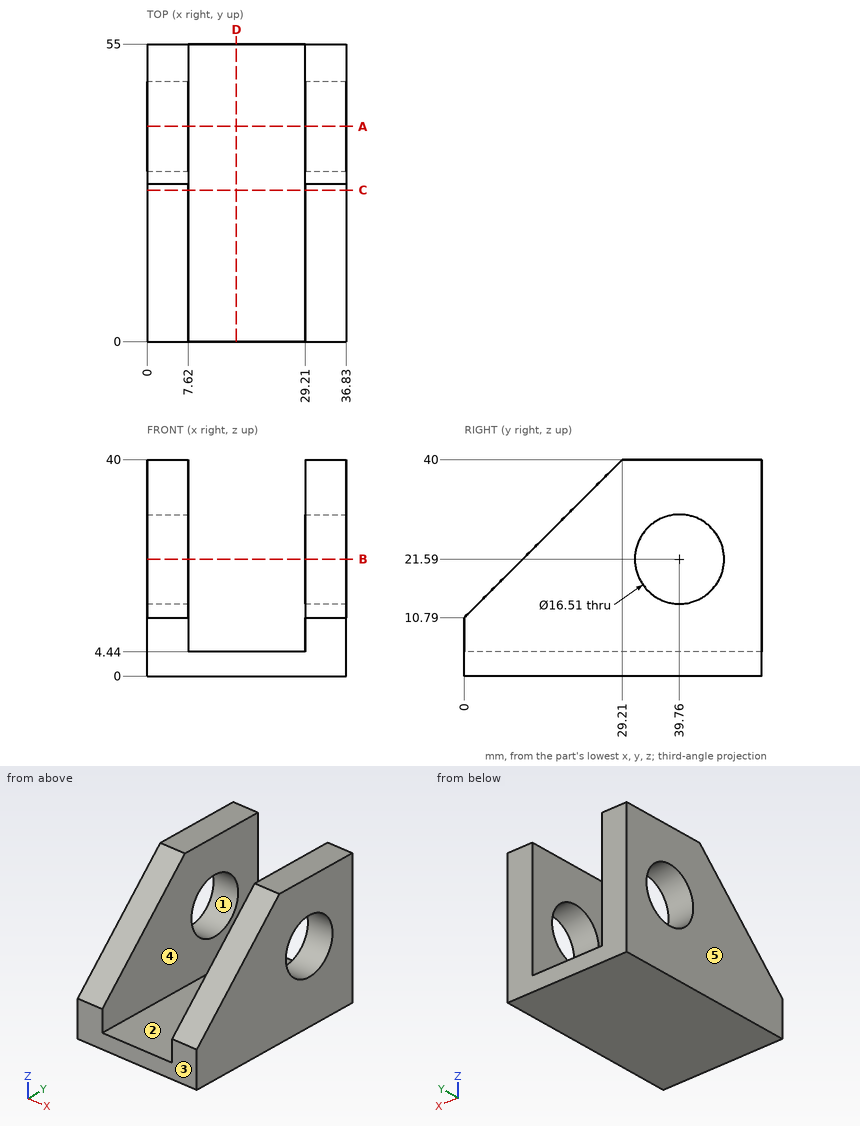
Can you work these out from the drawing? Everything is in mm from the part's minimum corner. A direction names the side the tool comes from. Give positions to 0.01 mm unless a question says otherwise; leave off trailing zeros. Loops run counter-clockwise (first coordinate to the right, second up) from the corner with the lowest first, then second, coordinate; pieces in that order, holes last. Notation, with made-up numbers: (37.25, -26) -> (93.25, -26) arc R12 ccw to (93.25, -16) -> close; hole circle Ø8 at (81.25, 86). An arc over 180 degrees is marked (long way). Return JSON: item names as keys, results as strings.
Item 1: If we section it at D-D on x = 16.5: List the corners of the cut face in (y, z) for me, plus the area to 3 significant figures.
Geometry results:
{"outline": "(0, 0) -> (55, 0) -> (55, 4.44) -> (0, 4.44) -> close", "area": "244 mm²"}
Item 2: If we section it at C-C on y = 28: List the corners of the cut face in (x, z) for me.
Geometry results:
{"outline": "(0, 0) -> (36.83, 0) -> (36.83, 38.79) -> (29.21, 38.79) -> (29.21, 4.44) -> (7.62, 4.44) -> (7.62, 38.79) -> (0, 38.79) -> close"}
Item 3: If we section it at B-B on z = 21.59: List the corners of the cut face in (x, y) for me (3 decimals), plus the area to 3 significant figures.
Geometry results:
{"outline": "(0, 10.8) -> (7.62, 10.8) -> (7.62, 31.505) -> (0, 31.505) -> close; (0, 48.015) -> (7.62, 48.015) -> (7.62, 55) -> (0, 55) -> close; (29.21, 10.8) -> (36.83, 10.8) -> (36.83, 31.505) -> (29.21, 31.505) -> close; (29.21, 48.015) -> (36.83, 48.015) -> (36.83, 55) -> (29.21, 55) -> close", "area": "422 mm²"}
Item 4: I'm going to push a flat-ended pin straight in: pin 1 (2 mm diameter, centred on x = 19, y = 6, fed in from +Z). Where does the tip first touch, or does it pass through?
Geometry results:
{"pin 1": "stops at z = 4.44"}
Item 5: We'd pull the mould along Y, two halves only. Please class the marked faces 1, 2 and 3: +Y half, -Y half, draft (parallel to the pull), parting line (faces both ways), or undercut.
Geometry results:
{"face 1": "undercut", "face 2": "draft", "face 3": "-Y half"}
Item 6: Which directions (+Z, -Z, +X, -X, +Y, -Y) give clear straight access to the entire face, cutting with the end or side of a thin tool? Please do the marked faces 4 and 5.
Geometry results:
{"face 4": "+Z, +Y, -Y", "face 5": "+Z, -Z, -X, +Y, -Y"}
Item 7: I need wall thicknesses on L1, parallel to Z at x = 31.5, y = 39.76 (3 decimals); L2, parallel to X at y = 26, z = 15.5; L3, parallel to Z at x = 26, y = 44. Which ranges of each line are inside material? Lowest first, please. Write a range as from..to.
Geometry results:
{"L1": "z = 0..13.335, 29.845..40", "L2": "x = 0..7.62, 29.21..36.83", "L3": "z = 0..4.44"}
Item 8: If we section it at A-A on y = 39.76: List the corners of the cut face in (x, z) for me (3 decimals), plus the area to 3 significant figures.
Geometry results:
{"outline": "(0, 0) -> (36.83, 0) -> (36.83, 13.335) -> (29.21, 13.335) -> (29.21, 4.44) -> (7.62, 4.44) -> (7.62, 13.335) -> (0, 13.335) -> close; (0, 29.845) -> (7.62, 29.845) -> (7.62, 40) -> (0, 40) -> close; (29.21, 29.845) -> (36.83, 29.845) -> (36.83, 40) -> (29.21, 40) -> close", "area": "454 mm²"}
